from build123d import *

# Parameters (mm, degrees)
F1_DEPTH = 1.27
F2_W     = 25.3899591044
F2_H     = 2.54
F3_DEPTH = 0.762
F4_DEPTH = 2.54
F5_DEPTH = 25.4


with BuildPart() as f1:
    # F0 (on Front) → F1 (new body, symmetric)
    with BuildSketch(Plane.XZ):
        with BuildLine():
            ThreePointArc((0, 0.508), (0.1487897552, 0.1487897552), (0.508, 0))
            Line((0.508, 0), (8.128, 0))
            Line((8.128, 0), (8.128, 2.54))
            Line((8.128, 2.54), (0.508, 2.54))
            ThreePointArc((0.508, 2.54), (0.1487897552, 2.3912102448), (0, 2.032))
            Line((0, 2.032), (0, 1.27))
            Line((0, 1.27), (0, 0.508))
        make_face()
        with BuildLine():
            ThreePointArc((2.3151677185, 1.27), (1.5279400395, 0.4827723211), (0.7407123606, 1.27))
            ThreePointArc((0.7407123606, 1.27), (1.5279400395, 2.0572276789), (2.3151677185, 1.27))
        make_face(mode=Mode.SUBTRACT)
        with BuildLine():
            ThreePointArc((2.3151677185, 1.27), (1.5279400395, 2.0572276789), (0.7407123606, 1.27))
            Line((0.7407123606, 1.27), (2.3151677185, 1.27))
        make_face()
        with BuildLine():
            Line((2.3151677185, 1.27), (0.7407123606, 1.27))
            ThreePointArc((0.7407123606, 1.27), (1.5279400395, 0.4827723211), (2.3151677185, 1.27))
        make_face()
    extrude(amount=F1_DEPTH, both=True)

    # F2 (on face) → F3 (join)
    with BuildSketch(Plane.YZ.offset(8.128)):
        with Locations((-1.2046988122, 1.27)):
            Rectangle(F2_W, F2_H)
    extrude(amount=-F3_DEPTH)

    # F0 (on Front) → F4 (join)
    with BuildSketch(Plane.XZ):
        with BuildLine():
            ThreePointArc((2.3151677185, 1.27), (1.5279400395, 2.0572276789), (0.7407123606, 1.27))
            Line((0.7407123606, 1.27), (2.3151677185, 1.27))
        make_face()
        with BuildLine():
            Line((2.3151677185, 1.27), (0.7407123606, 1.27))
            ThreePointArc((0.7407123606, 1.27), (1.5279400395, 0.4827723211), (2.3151677185, 1.27))
        make_face()
    extrude(amount=F4_DEPTH)

    # F0 (on Front) → F5 (cut)
    with BuildSketch(Plane.XZ):
        with BuildLine():
            ThreePointArc((2.3151677185, 1.27), (1.5279400395, 2.0572276789), (0.7407123606, 1.27))
            Line((0.7407123606, 1.27), (2.3151677185, 1.27))
        make_face()
        with BuildLine():
            Line((2.3151677185, 1.27), (0.7407123606, 1.27))
            ThreePointArc((0.7407123606, 1.27), (1.5279400395, 0.4827723211), (2.3151677185, 1.27))
        make_face()
    extrude(amount=-F5_DEPTH, mode=Mode.SUBTRACT)


solid = f1.part
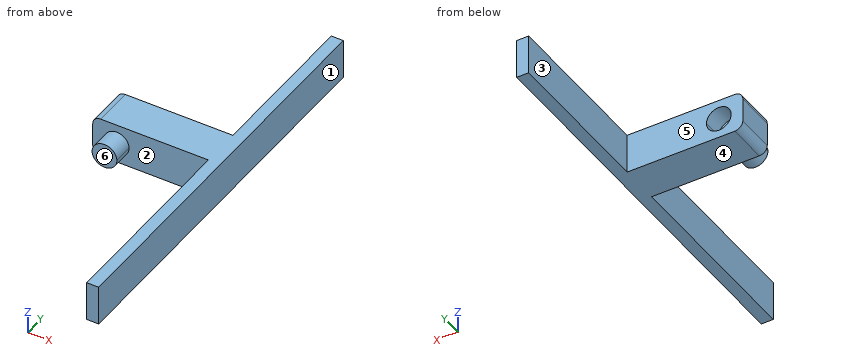
Geometry: final body of the model. Coordinates: model frame, mm. Face numbers are marked on the shaded views. A direction names the side the tool comes from. Give positions to 0.01 mm unless a question says otherwise; leave off trailing zeros. Order: outer loops, then holes, each group sorted by start corner. A loop starts at its lowest first (then second) coordinate and runs counter-clockwise, first axis right, second up. Notation, with made-up numbers: (-35.75, 62) -> (-0.75, 62) arc R25 cw to (-0.75, 85) -> close; hole circle Ø9 at (72.5, 78.5). An arc over 180 degrees is marked (long way). Write each question's results on one line, items separated by ' | '.
1) First-contact query: pin 1 Ø1.3 at (x, z) = (1.5, 1) entering from -Y; pin 2 Ø1.3 at (x, z) = (5, 1) entering from +Y. Flat tips, straight axial feed; report the tip coordinate or a pass-through.
Geometry says:
pin 1: stops at y = -2.54 | pin 2: stops at y = 1.27
2) Set-up query: the marked faces 4, 5 and 6. Return all of +Z, -Z, +X, -X, +Y, -Y with unobstructed straight access to the full face (end or side cutting, diameter ignored); none if empty.
Geometry says:
face 4: -Z, +X, -X, +Y, -Y | face 5: +Z, -Z, -X, +Y | face 6: +Z, -Z, -X, -Y
3) Cut plane B-B (x = 4.25). Output: boundary loops of the cut face in (y, z), and give its area (3 significant figures).
Geometry says:
outline: (-1.27, 0) -> (1.27, 0) -> (1.27, 2.54) -> (-1.27, 2.54) -> close | area: 6.45 mm²
4) Draft query along X for the marked faces 1, 2 and 3. Return one class per face: released by +X, released by -X, zero draft, split by the parting line, or undercut.
Geometry says:
face 1: released by +X | face 2: undercut | face 3: released by -X
5) Cut plane A-A (y = -7.5). Output: boundary loops of the cut face in (x, z), and give its area (3 significant figures).
Geometry says:
outline: (7.37, 0) -> (8.13, 0) -> (8.13, 2.54) -> (7.37, 2.54) -> close | area: 1.94 mm²
6) Line query: line 1 along Y through (x, z) = (3.5, 1.75); line 2 along X through (y, z) = (-11, 1.95); line 3 along Y through (x, z) = (2, 1.65). Output: solid intervals per line, ascending.
Geometry says:
line 1: y = -1.27 to 1.27 | line 2: x = 7.37 to 8.13 | line 3: y = -2.54 to 0
